```python
from build123d import *

# Parameters (mm, degrees)
SKETCH1_W           = 100
SKETCH1_H           = 84
BOSS_EXTRUDE1_DEPTH = 6
SKETCH2_W           = 100
SKETCH2_H           = 44
BOSS_EXTRUDE2_DEPTH = 6
SKETCH3_W           = 100
SKETCH3_H           = 84
BOSS_EXTRUDE3_DEPTH = 31
SKETCH4_W           = 30
SKETCH4_H           = 5.699357211
CUT_EXTRUDE1_DEPTH  = 30
SKETCH5_R           = 2
CUT_EXTRUDE2_DEPTH  = 113.805141727
SKETCH6_W           = 87.5
SKETCH6_H           = 26
CUT_EXTRUDE3_DEPTH  = 15
SKETCH7_R           = 2
CUT_EXTRUDE4_DEPTH  = 113.805141727
SKETCH8_W           = 20
SKETCH8_H           = 14.276989135
CUT_EXTRUDE5_DEPTH  = 15


with BuildPart() as part:
    # Sketch1 → Boss-Extrude1 (new body)
    with BuildSketch(Plane(origin=(0, 0, 0), x_dir=(1, 0, 0), z_dir=(0, 1, 0))):
        Rectangle(SKETCH1_W, SKETCH1_H)
    extrude(amount=BOSS_EXTRUDE1_DEPTH)

    # Sketch2 → Boss-Extrude2 (add)
    with BuildSketch(Plane(origin=(0, 6, 0), x_dir=(1, 0, 0), z_dir=(0, 1, 0))):
        with Locations((0, -1)):
            Rectangle(SKETCH2_W, SKETCH2_H)
    extrude(amount=BOSS_EXTRUDE2_DEPTH)

    # Sketch3 → Boss-Extrude3 (add)
    with BuildSketch(Plane.XZ):
        Rectangle(SKETCH3_W, SKETCH3_H)
    extrude(amount=BOSS_EXTRUDE3_DEPTH)

    # Sketch4 → Cut-Extrude1 (cut)
    with BuildSketch(Plane(origin=(0, 0, -42), x_dir=(-1, 0, 0), z_dir=(0, 0, -1))):
        with Locations((0, -2.849678606)):
            Rectangle(SKETCH4_W, SKETCH4_H)
    extrude(amount=-CUT_EXTRUDE1_DEPTH, mode=Mode.SUBTRACT)

    # Sketch5 → Cut-Extrude2 (cut, through all)
    with BuildSketch(Plane.ZY.offset(50)):
        with Locations((37.5, 1.5)):
            Circle(SKETCH5_R)
    extrude(amount=-CUT_EXTRUDE2_DEPTH, mode=Mode.SUBTRACT)

    # Sketch6 → Cut-Extrude3 (cut)
    with BuildSketch(Plane(origin=(0, 6, 0), x_dir=(1, 0, 0), z_dir=(0, 1, 0))):
        with Locations((0, -41)):
            Rectangle(SKETCH6_W, SKETCH6_H)
    extrude(amount=-CUT_EXTRUDE3_DEPTH, mode=Mode.SUBTRACT)

    # Sketch7 → Cut-Extrude4 (cut, through all)
    with BuildSketch(Plane(origin=(50, 0, 0), x_dir=(0, 0, -1), z_dir=(1, 0, 0))):
        with Locations((36.5, 0.5)):
            Circle(SKETCH7_R)
    extrude(amount=-CUT_EXTRUDE4_DEPTH, mode=Mode.SUBTRACT)

    # Sketch8 → Cut-Extrude5 (cut)
    with BuildSketch(Plane(origin=(0, 6, 0), x_dir=(1, 0, 0), z_dir=(0, 1, 0))):
        with Locations((-35, 34.861505433)):
            Rectangle(SKETCH8_W, SKETCH8_H)
        with Locations((35, 34.861505433)):
            Rectangle(SKETCH8_W, SKETCH8_H)
    extrude(amount=-CUT_EXTRUDE5_DEPTH, mode=Mode.SUBTRACT)


solid = part.part
```
Geometry check sheet. Reference: the model listing, model coordinates, mm. A direction names the side the tool comes from. Give positions to 0.01 mm unless a question says otherwise; leave off trailing zeros. Order: outer loops, then holes, each group sorted by start corner. A loop starts at its lowest first (then second) coordinate and runs counter-clockwise, first axis right, second up. Notation, with made-up numbers: (-13, 6) - (-8, 6) arc R15 cw to (-8, 20) - close; hole circle Ø5 at (76.5, 14). An arc over 180 degrees is marked (long way). Answer in a Markdown table with one row per item. Add a question column.
Q1. Mould release check, pull along X, two halves, no side actions. Record for faces 5 (the flat face through (35, -9, -35)), 6 (the cylindrical face through (-47.465, 0.588, -34.502)): pulls with the +X half, pulls with the -X half, needs draft (parallel to the pull), parting line crosses it, or undercut.
Q2. Material ranges on probe 1 along X at (y, z) = (3, -38); probe 2 along Z at (x, y) = (48, 0); probe 3 along Y at (x, z) = (-4.5, -36.5), recorded low to high. Write a range as from..to.
Q3. Cross-section at A-A, the plane z = 37.5. Enter the section's corners in (x, y).
Q4. Cross-section at B-B, the plane z = -36.5. Enter the section's corners in (x, y).
Q5. Cross-section at D-D, the plane x = 27. Enter the section's corners in (y, z).
Q6. Cross-section at C-C, the plane y = -7. Enter the section's corners in (x, z).
Q7. Tool access check on faces 1 (the flat face through (-1, 6, -32)), 2 (the flat face through (-1, -9, 35)), 3 (the flat face through (0, -5.699, -27)), 4 (the flat face through (45, -1.4, -34.8)). Record the directions out of +Z, -Z, +X, -X, +Y, -Y that give a thin tool (end or side, any length) a straight path to the whole face; none if there is none.
Q8. Gauge pin test, flat ends, axial feed: pin 1 (21 mm diameter, centred on x = 10.5, z = 35.5, fed in from +Y); pin 2 (7 mm diameter, centred on x = -32.5, z = -34, fed in from +Y); pin 3 (12 mm diameter, centred on x = 39.5, y = -2.5, fed in from -Z); pin 4 (1.7 mm diameter, centred on x = 7, y = -3.5, fed in from -Z). Record the tip position at first contact, or that the pin passes through.
Check values:
| question | item | result |
|---|---|---|
| 1 | face 5 | undercut |
| 1 | face 6 | needs draft |
| 2 | probe 1 | x = -50..-45, -25..25, 45..50 |
| 2 | probe 2 | z = -42..-38.44, -34.56..36.18, 38.82..42 |
| 2 | probe 3 | y = -31..-5.7, 2.5..6 |
| 3 | outline | (-50, -31) - (50, -31) - (50, -0.5) - (43.75, -0.5) - (43.75, -9) - (-43.75, -9) - (-43.75, -0.5) - (-50, -0.5) - close; (-50, 3.5) - (-43.75, 3.5) - (-43.75, 6) - (-50, 6) - close; (43.75, 3.5) - (50, 3.5) - (50, 6) - (43.75, 6) - close |
| 4 | outline | (-50, -31) - (50, -31) - (50, -1.5) - (45, -1.5) - (45, -9) - (25, -9) - (25, -1.5) - (15, -1.5) - (15, -5.7) - (-15, -5.7) - (-15, -1.5) - (-25, -1.5) - (-25, -9) - (-45, -9) - (-45, -1.5) - (-50, -1.5) - close; (-50, 2.5) - (-45, 2.5) - (-45, 6) - (-50, 6) - close; (-25, 2.5) - (25, 2.5) - (25, 6) - (-25, 6) - close; (45, 2.5) - (50, 2.5) - (50, 6) - (45, 6) - close |
| 5 | outline | (-31, -42) - (-9, -42) - (-9, -27.72) - (6, -27.72) - (6, -21) - (12, -21) - (12, 23) - (6, 23) - (6, 28) - (-9, 28) - (-9, 42) - (-31, 42) - close |
| 6 | outline | (-50, -42) - (-45, -42) - (-45, -27.72) - (-25, -27.72) - (-25, -42) - (25, -42) - (25, -27.72) - (45, -27.72) - (45, -42) - (50, -42) - (50, 42) - (43.75, 42) - (43.75, 28) - (-43.75, 28) - (-43.75, 42) - (-50, 42) - close |
| 7 | face 1 | -Z, +X, -X, +Y |
| 7 | face 2 | +Z, +Y |
| 7 | face 3 | -Z |
| 7 | face 4 | -Z, +Y |
| 8 | pin 1 | stops at y = 6 |
| 8 | pin 2 | stops at y = -9 |
| 8 | pin 3 | stops at z = -42 |
| 8 | pin 4 | stops at z = -12 |
